Work out the finished part from the listing and answer in its coordinate system (mm). Face numbers are marked on the shaded views. A direction names the side the tool comes from. Coordinates: 2 decimals unless noted, no trailing zeros. Loops run counter-clockwise (first coordinate to the right, second up) from the corner with the lowest first, then second, coordinate; pieces in that order, holes last. Notation, with made-up numbers: (27, 69.5) -> (45, 69.5) arc R30 cw to (45, 93.5) -> close; hole circle Ø1 at (24.5, 13). An arc over 180 degrees is marked (long way). Use a Markdown table: item, result.
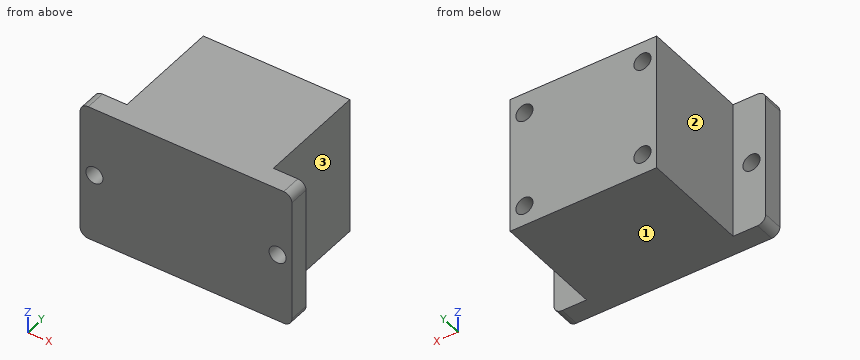
from build123d import *

# Parameters (mm, degrees)
SKETCH_1_W          = 52
SKETCH_1_H          = 34
SKETCH_1_R          = 2.1
EXTRUDE_1_DEPTH     = 5
SKETCH_2_W          = 36
SKETCH_2_H          = 34
EXTRUDE_2_DEPTH     = 27
SKETCH_3_R          = 2.1
CUT_EXTRUDE_1_DEPTH = 10
FILLET_1_R          = 2
FILLET_2_R          = 2
FILLET_3_R          = 2
FILLET_4_R          = 2


with BuildPart() as part:
    # 草图1 → 凸台-拉伸1 (new body)
    with BuildSketch(Plane(origin=(0, 0, 0), x_dir=(1, 0, 0), z_dir=(0, 1, 0))):
        with Locations((1, 0)):
            Rectangle(SKETCH_1_W, SKETCH_1_H)
        with Locations(Location((-21.5, 0, 0), (0, 0, 270))):
            Circle(SKETCH_1_R, mode=Mode.SUBTRACT)
        with Locations(Location((23.5, 0, 0), (0, 0, 90))):
            Circle(SKETCH_1_R, mode=Mode.SUBTRACT)
    extrude(amount=EXTRUDE_1_DEPTH)

    # 草图2 → 凸台-拉伸2 (add)
    with BuildSketch(Plane(origin=(0, 5, 0), x_dir=(1, 0, 0), z_dir=(0, 1, 0))):
        with Locations((1, 0)):
            Rectangle(SKETCH_2_W, SKETCH_2_H)
    extrude(amount=EXTRUDE_2_DEPTH)

    # 草图3 → 切除-拉伸1 (cut)
    with BuildSketch(Plane(origin=(0, 32, 0), x_dir=(1, 0, 0), z_dir=(0, 1, 0))):
        with Locations(Location((-13.5, 12, 0), (0, 0, 270))):
            Circle(SKETCH_3_R)
        with Locations(Location((15.5, 12, 0), (0, 0, 270))):
            Circle(SKETCH_3_R)
        with Locations(Location((15.5, -12, 0), (0, 0, 270))):
            Circle(SKETCH_3_R)
        with Locations(Location((-13.5, -12, 0), (0, 0, 270))):
            Circle(SKETCH_3_R)
    extrude(amount=-CUT_EXTRUDE_1_DEPTH, mode=Mode.SUBTRACT)

    # 圆角1
    fillet_1_edges = [part.edges().sort_by_distance(p)[0] for p in [
        (-25, 2.5, -17),
    ]]
    fillet(fillet_1_edges, radius=FILLET_1_R)

    # 圆角2
    fillet_2_edges = [part.edges().sort_by_distance(p)[0] for p in [
        (-25, 2.5, 17),
    ]]
    fillet(fillet_2_edges, radius=FILLET_2_R)

    # 圆角3
    fillet_3_edges = [part.edges().sort_by_distance(p)[0] for p in [
        (27, 2.5, 17),
    ]]
    fillet(fillet_3_edges, radius=FILLET_3_R)

    # 圆角4
    fillet_4_edges = [part.edges().sort_by_distance(p)[0] for p in [
        (27, 2.5, -17),
    ]]
    fillet(fillet_4_edges, radius=FILLET_4_R)


solid = part.part
Q1. Section B-B on y = 2.5 is taken. Determine the outline of the cut face in (x, z).
Solved:
| item | result |
|---|---|
| outline | (-25, -15) arc R2 ccw to (-23, -17) -> (25, -17) arc R2 ccw to (27, -15) -> (27, 15) arc R2 ccw to (25, 17) -> (-23, 17) arc R2 ccw to (-25, 15) -> close; hole circle Ø4.2 at (-21.5, 0); hole circle Ø4.2 at (23.5, 0) |
Q2. Section A-A on x = -21.5 is taken. Determine the outline of the cut face in (y, z).
Solved:
| item | result |
|---|---|
| outline | (0, -17) -> (5, -17) -> (5, -2.1) -> (0, -2.1) -> close; (0, 2.1) -> (5, 2.1) -> (5, 17) -> (0, 17) -> close |
Q3. Consider line 1 (X direction, y = 25, z = -12); line 2 (Z direction, x = 23.5, y = 2.45); line 3 (X direction, y = 23, z = -11). Determine where each line is inside the solid, lowest interval first. Write a range as [from, to].
Solved:
| item | result |
|---|---|
| line 1 | [-17, -15.6], [-11.4, 13.4], [17.6, 19] |
| line 2 | [-17, -2.1], [2.1, 17] |
| line 3 | [-17, -15.35], [-11.65, 13.65], [17.35, 19] |
Q4. Section D-D on y = 26 is taken. Determine the outline of the cut face in (x, z), and give its area (3 significant figures).
Solved:
| item | result |
|---|---|
| outline | (-17, -17) -> (19, -17) -> (19, 17) -> (-17, 17) -> close; hole circle Ø4.2 at (-13.5, -12); hole circle Ø4.2 at (-13.5, 12); hole circle Ø4.2 at (15.5, -12); hole circle Ø4.2 at (15.5, 12) |
| area | 1,170 mm² |
Q5. Section C-C on z = 0 is taken. Determine the outline of the cut face in (x, y), and give its area (3 significant figures).
Solved:
| item | result |
|---|---|
| outline | (-25, 0) -> (-23.6, 0) -> (-23.6, 5) -> (-25, 5) -> close; (-19.4, 0) -> (21.4, 0) -> (21.4, 5) -> (19, 5) -> (19, 32) -> (-17, 32) -> (-17, 5) -> (-19.4, 5) -> close; (25.6, 0) -> (27, 0) -> (27, 5) -> (25.6, 5) -> close |
| area | 1,190 mm² |
Q6. Given pin 1 Ø13.5 at (y, z) = (19.5, -7) entering from -X; pin 2 Ø1.3 at (x, z) = (-13, 12.5) entering from +Y; pin 3 Ø3.5 at (x, z) = (23.5, 0) entering from +Y; pin 4 Ø4 at (x, z) = (-22, -3) entering from +Y, each flat-ended and moving along its own axis, determine where each tip first touches the part or whether it passes through.
Solved:
| item | result |
|---|---|
| pin 1 | x = -17 |
| pin 2 | y = 22 |
| pin 3 | through |
| pin 4 | y = 5 |
Q7. For the marked faces 1, 2 and 3, determine the directions among +Z, -Z, +X, -X, +Y, -Y from which every point of the face is accessible in a straight line to the end or side of a thin tool.
Solved:
| item | result |
|---|---|
| face 1 | -Z, +X, -X, +Y, -Y |
| face 2 | +Z, -Z, -X, +Y |
| face 3 | +Z, -Z, +X, +Y |
